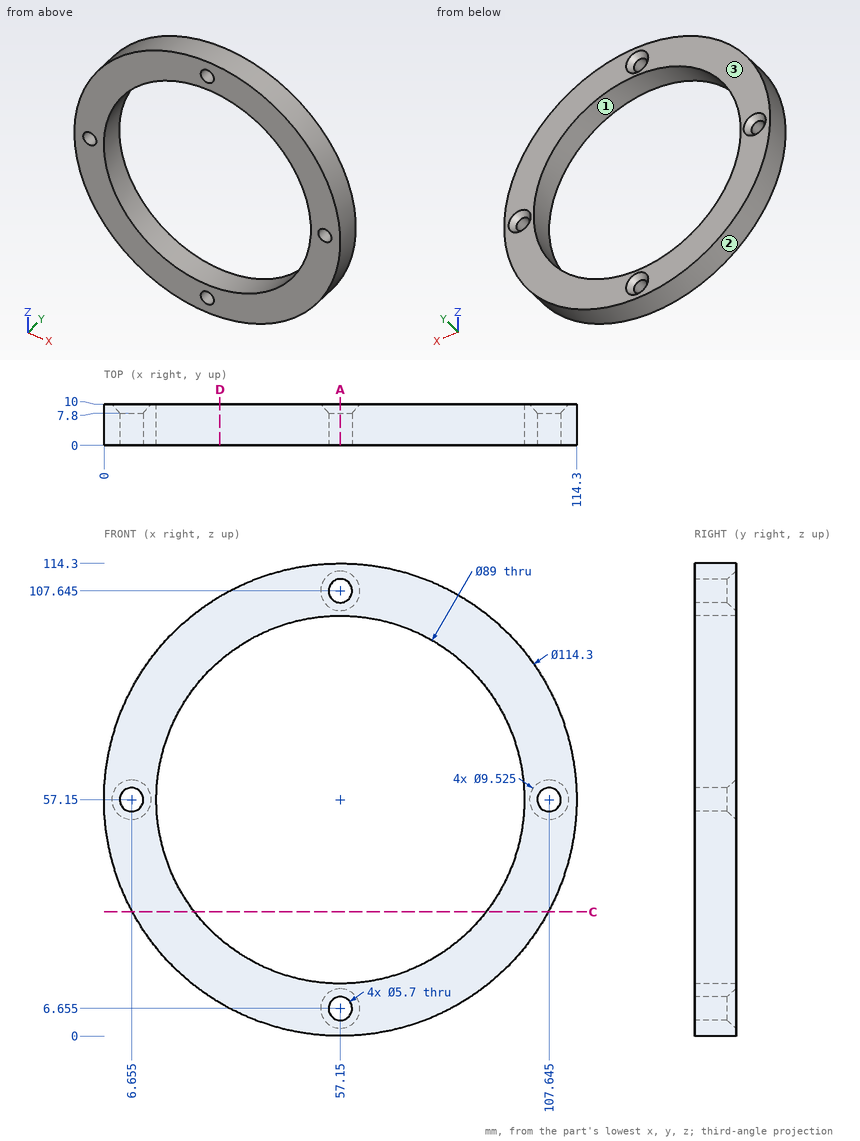
Verification items for this drawing (mm, ordinates from the low corner). Round coordinates to 2 decimals unless told otherwise and drop trailing zeros. Loops run counter-clockwise (first coordinate to the right, second up) from the corner with the lowest first, then second, coordinate; pieces in that order, holes last. Notation, with made-up numbers: (58, 3) -> (90, 3) arc R31 cw to (90, 30) -> close; hole circle Ø4 at (3.25, 55.5). An arc over 180 degrees is marked (long way). Write item = value, one per line. Start each with the question number.
1) Sectioned sample at C-C, the plane z = 30. Record the cut outline in (x, y), plus the area to 3 significant figures.
2) Release check for a two-part mould opening along X. For the marked faces 1, 2 and 3 record: released by +X, released by -X, zero draft, split by the parting line, or undercut.
3) Gauge pin test, flat ends, axial feed: pin 1 Ø5 at (x, z) = (107.65, 57.15) entering from -Y; pin 2 Ø1 at (x, y) = (86.5, 3.5) entering from +Z; pin 3 Ø1 at (y, z) = (8.5, 60.5) entering from +X; pin 4 Ø6 at (y, z) = (6, 70.5) entering from -X (3 decimals). Record the tip position at first contact, or that the pin passes through.
4) Thickness scan on probe 1 along Z at (x, y) = (59, 3.5); probe 2 along Z at (x, y) = (74, 7); probe 3 along X at (y, z) = (2, 97.5) (1 decimal). Record the ranges inside material, lowest first.
5) Sectioned sample at A-A, the plane x = 57.15. State how many separate pieces and enclosed holes the cut face has, plus the area to 3 significant figures.
6) Sectioned sample at D-D, the plane x = 28. Record the cut outline in (y, z).
Results are:
q1.outline = (6.86, 0) -> (21.89, 0) -> (21.89, 10) -> (6.86, 10) -> close; (92.41, 0) -> (107.44, 0) -> (107.44, 10) -> (92.41, 10) -> close
q1.area = 301 mm^2
q2.face_1 = undercut
q2.face_2 = split by the parting line
q2.face_3 = zero draft
q3.pin_1 = through
q3.pin_2 = 106.48
q3.pin_3 = 114.23
q3.pin_4 = 0.945
q4.probe_1 = 0.03 to 4.49, 8.82 to 12.69, 101.61 to 105.48, 109.81 to 114.27
q4.probe_2 = 2.54 to 15.96, 98.34 to 111.76
q4.probe_3 = 16.7 to 38.4, 75.9 to 97.6
q5.separate_pieces = 4
q5.enclosed_holes = 0
q5.area = 131 mm^2
q6.outline = (0, 7.99) -> (10, 7.99) -> (10, 23.53) -> (0, 23.53) -> close; (0, 90.77) -> (10, 90.77) -> (10, 106.31) -> (0, 106.31) -> close
